Could you check a few things on this drawing? It's one solid part, dimensions in mm from its lowest x, y, z. A direction names the side the tool comes from. Give positions to 0.01 mm unless a question says otherwise; leave off trailing zeros. Order: outer loops, then holes, each group sorted by start corner. A loop starts at its lowest first (then second) coordinate and runs counter-clockwise, first axis right, second up. Notation, with made-up numbers: (65, -19) -> (80, -19) arc R25 cw to (80, 10) -> close; hole circle Ø7 at (40.5, 3.5). An arc over 180 degrees is marked (long way). Answer as CSV lines item,"result".
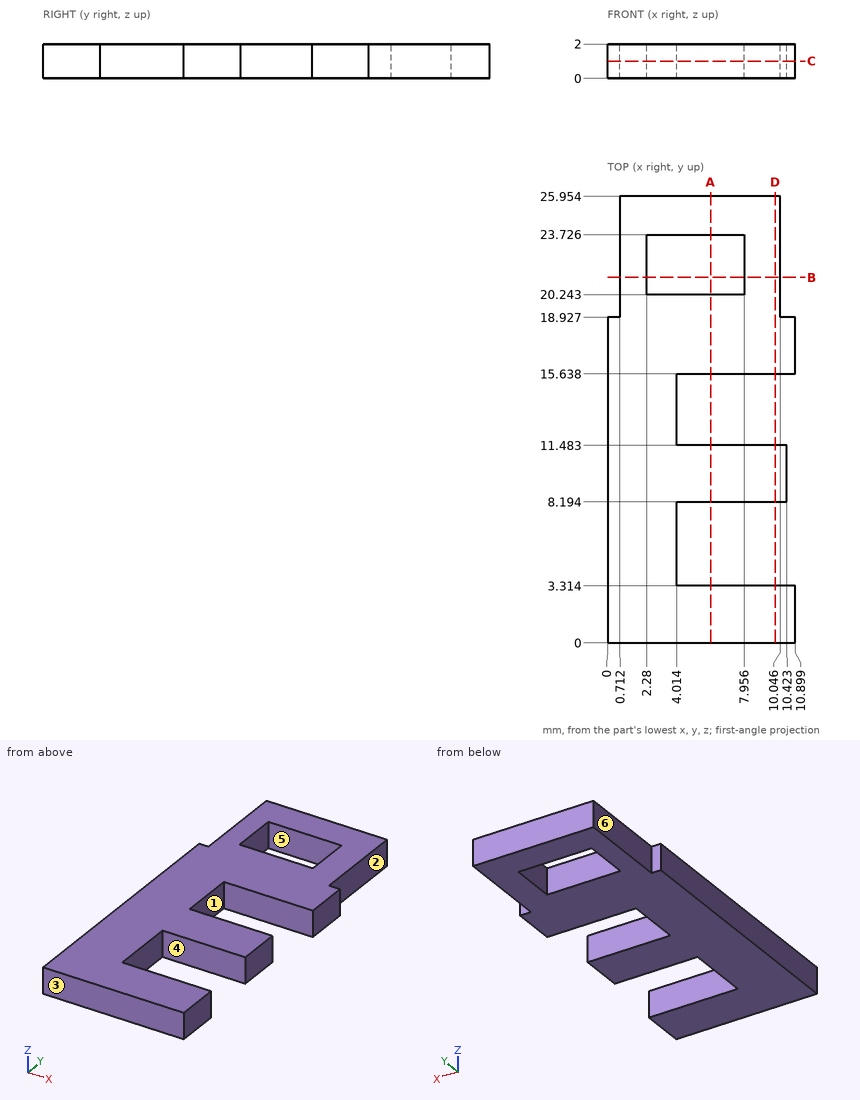
Item 1: Please list where these lines run through material, in increasing order: line 1 along Y through (x, z) = (7.75, 1.1) (1 decimal); line 2 along Y through (x, z) = (10.25, 1.4); line 3 along X through (y, z) = (20.75, 1.2) (1 decimal).
Numbers:
line 1,"y = 0 to 3.3, 8.2 to 11.5, 15.6 to 20.2, 23.7 to 26"
line 2,"y = 0 to 3.31, 8.19 to 11.48, 15.64 to 18.93"
line 3,"x = 0.7 to 2.3, 8 to 10"
Item 2: Imagine slicing it at B-B, the plane y = 21.25. Please give me the cut outline in (x, z) (1 decimal).
Numbers:
outline,"(0.7, 0) -> (2.3, 0) -> (2.3, 2) -> (0.7, 2) -> close; (8, 0) -> (10, 0) -> (10, 2) -> (8, 2) -> close"
Item 3: For the marked faces 4, 5 and 6, which set-ups out of +Z, -Z, +X, -X, +Y, -Y let a thin tool reach every point of the face, with its end or its side?
Numbers:
face 4,"+Z, -Z, +X"
face 5,"+Z, -Z"
face 6,"+Z, -Z, -X, +Y"
Item 4: Imagine slicing it at C-C, the plane z = 1. Please give me the cut outline in (x, y) (1 decimal).
Numbers:
outline,"(0, 0) -> (10.9, 0) -> (10.9, 3.3) -> (4, 3.3) -> (4, 8.2) -> (10.4, 8.2) -> (10.4, 11.5) -> (4, 11.5) -> (4, 15.6) -> (10.9, 15.6) -> (10.9, 18.9) -> (10, 18.9) -> (10, 26) -> (0.7, 26) -> (0.7, 18.9) -> (0, 18.9) -> close; hole (2.3, 20.2) -> (8, 20.2) -> (8, 23.7) -> (2.3, 23.7) -> close"
Item 5: We'd pull the mould along Y, two halves only. Please class the marked faces 1, 2 and 3: released by +Y, released by -Y, zero draft, split by the parting line, or undercut.
Numbers:
face 1,"undercut"
face 2,"zero draft"
face 3,"released by -Y"
Item 6: Imagine slicing it at D-D, the plane x = 9.75. Please give me the cut outline in (y, z) (1 decimal).
Numbers:
outline,"(0, 0) -> (3.3, 0) -> (3.3, 2) -> (0, 2) -> close; (8.2, 0) -> (11.5, 0) -> (11.5, 2) -> (8.2, 2) -> close; (15.6, 0) -> (26, 0) -> (26, 2) -> (15.6, 2) -> close"
Item 7: For pin 1 (6 mm diameter, centred on x = 8.5, y = 18, fed in from -Z); pin 2 (0.6 mm diameter, centred on y = 21.5, z = 1.5, fed in from -X); pin 3 (2 mm diameter, centred on x = 8, y = 14.5, fed in from +Z); pin 4 (0.7 mm diameter, centred on x = 10.5, z = 1, fed in from +Y), each with a flat end and sliding along its axis, tell me the tip position at first contact or that it passes through.
Numbers:
pin 1,"stops at z = 0"
pin 2,"stops at x = 0.71"
pin 3,"passes through"
pin 4,"stops at y = 18.93"
Item 8: Imagine slicing it at A-A, the plane x = 6. Please give me the cut outline in (y, z) (1 decimal).
Numbers:
outline,"(0, 0) -> (3.3, 0) -> (3.3, 2) -> (0, 2) -> close; (8.2, 0) -> (11.5, 0) -> (11.5, 2) -> (8.2, 2) -> close; (15.6, 0) -> (20.2, 0) -> (20.2, 2) -> (15.6, 2) -> close; (23.7, 0) -> (26, 0) -> (26, 2) -> (23.7, 2) -> close"
